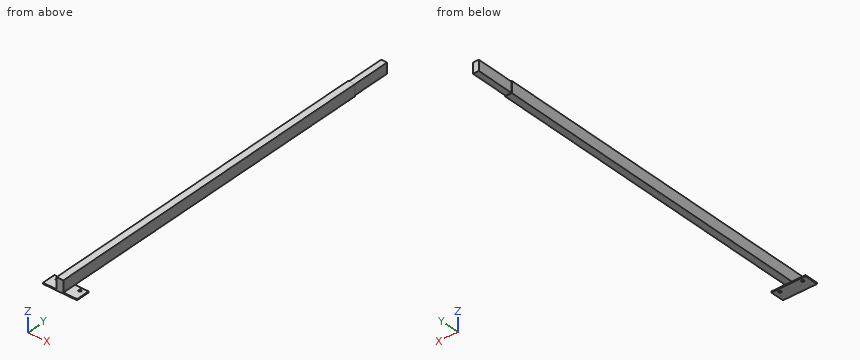
from build123d import *

# Parameters (mm, degrees)
F0_W     = 26
F0_H     = 46
F1_DEPTH = 170
F2_W     = 30
F2_H     = 50
F3_DEPTH = 1520
F4_W     = 60
F4_H     = 60
F4_R     = 6
F5_DEPTH = 5


with BuildPart() as f1:
    # F0 (on Front) → F1 (new body)
    with BuildSketch(Plane.XZ):
        Rectangle(F0_W, F0_H)
    extrude(amount=F1_DEPTH)

    # F2 (on face) → F3 (join)
    with BuildSketch(Plane.XZ.offset(170)):
        Rectangle(F2_W, F2_H)
    extrude(amount=F3_DEPTH)

    # F4 (on face) → F5 (join)
    with BuildSketch(Plane(origin=(0, 0, -25), x_dir=(1, 0, 0), z_dir=(0, 0, -1))):
        Polygon((15, 1690), (-15, 1690), (-15, 1630), (15, 1630), (15, 1645), align=None)
        with Locations((-45, 1660)):
            Rectangle(F4_W, F4_H)
        with Locations((-50, 1645)):
            Circle(F4_R, mode=Mode.SUBTRACT)
        with BuildLine():
            ThreePointArc((56, 1645), (50, 1651), (44, 1645))
            ThreePointArc((44, 1645), (50, 1639), (56, 1645))
        make_face()
        Polygon((75, 1690), (15, 1690), (15, 1645), (15, 1630), (75, 1630), align=None)
        with BuildLine():
            ThreePointArc((56, 1645), (50, 1639), (44, 1645))
            ThreePointArc((44, 1645), (50, 1651), (56, 1645))
        make_face(mode=Mode.SUBTRACT)
    extrude(amount=F5_DEPTH)


solid = f1.part
Can you work these out from the model? Positions are in its coordinate system, mm. Coordinates: 2 decimals unless noted, no trailing zeros. Order: outer loops, then holes, each group sorted by start corner. A loop starts at its lowest first (then second) coordinate and runs counter-clockwise, first axis right, second up. Notation, with made-up numbers: M 77.25,10 L 87.25,10 A19 cw 87.25,39 Z; hole C -7,86.5 d7. An arc over 180 degrees is marked long. Write item = value, one per line.
(1) I need wall thicknesses on line 1 along X through (y, z) = (-1645, -28); line 2 along Y through (x, z) = (50, -28); line 3 along X through (y, z) = (-441, -22.5). Which ranges of each line are inside material? Lowest first, please. Write a range as [from, to].
Results are:
line_1 = [-75, -56], [-44, 44], [56, 75]
line_2 = [-1690, -1651], [-1639, -1630]
line_3 = [-15, 15]
(2) Suppose I cut it at A-A on z = 13. Please give me the cut outline in (x, y), plus the area to 3 significant figures.
Results are:
outline = M -15,-1690 L 15,-1690 L 15,-170 L 13,-170 L 13,0 L -13,0 L -13,-170 L -15,-170 Z
area = 50,000 mm2
(3) For pin 1 Ø14 at (y, z) = (-92.5, 7.5) entering from +X; pin 2 Ø21 at (x, y) = (5.5, -117) entering from -Z; pin 3 Ø15 at (x, z) = (-6, 5) entering from +Y; pin 4 Ø5 at (y, z) = (-1465, -8) entering from -X, each with a flat end and sliding along its axis, tell me the tip position at first contact or that it passes through.
Results are:
pin_1 = 13
pin_2 = -23
pin_3 = 0
pin_4 = -15
(4) Suppose I cut it at B-B on y = -535.5. Please give me the cut outline in (x, z), plus the area to 3 significant figures.
Results are:
outline = M -15,-25 L 15,-25 L 15,25 L -15,25 Z
area = 1,500 mm2
